Work out the finished part from the listing and answer in its coordinate system (mm). A direction names the side the tool comes from. Coordinates: 2 decimals unless noted, no trailing zeros. Loops run counter-clockwise (first coordinate to the right, second up) from the corner with the lowest first, then second, coordinate; pieces in that order, holes last. Notation, with made-up numbers: M 9,-7.5 L 20,-7.5 A10 cw 20,3.5 Z; hole C 1,78 d9. An arc over 180 degrees is marked long. Write each question's results on one line, items separated by ' | '.
```python
from build123d import *

# Parameters (mm, degrees)
SKETCH1_W              = 25
SKETCH1_H              = 40
BOSS_EXTRUDE1_DEPTH    = 1.6
SKETCH2_W              = 5
SKETCH2_H              = 5
BOSS_EXTRUDE2_DEPTH    = 0.5
SKETCH3_W              = 5
SKETCH3_H              = 3
BOSS_EXTRUDE3_DEPTH    = 2
SKETCH4_R              = 0.95
BOSS_EXTRUDE6_DEPTH    = 2.75
FILLET2_R              = 0.75
LPATTERN2_COUNT        = 3
LPATTERN2_PITCH        = 4
FILLET2_OF_LPATTERN2_R = 0.75
BOSS_EXTRUDE7_DEPTH    = 2.75
SKETCH6_RX             = 1.75
SKETCH6_RY             = 1
BOSS_EXTRUDE8_DEPTH    = 3.5
SKETCH7_W              = 8
SKETCH7_H              = 8
SKETCH7_W_2            = 2.174963518
SKETCH7_H_2            = 1.544625232
SKETCH7_W_3            = 2.304661065
SKETCH7_H_3            = 2.304661065
SKETCH7_W_4            = 1.577304609
SKETCH7_H_4            = 2.386179735
BOSS_EXTRUDE9_DEPTH    = 0.1
SKETCH8_W              = 2.304661065
SKETCH8_H              = 2.304661065
SKETCH8_W_2            = 1.577304609
SKETCH8_H_2            = 2.386179735
SKETCH8_W_3            = 2.174963518
SKETCH8_H_3            = 1.544625232
BOSS_EXTRUDE10_DEPTH   = 1
SKETCH9_W              = 2.75
SKETCH9_H              = 7
BOSS_EXTRUDE11_DEPTH   = 1.5
SKETCH10_W             = 3
SKETCH10_H             = 1
BOSS_EXTRUDE12_DEPTH   = 5
LPATTERN3_COUNT        = 2
LPATTERN3_PITCH        = 17
SKETCH11_W             = 0.854141563
SKETCH11_H             = 2.134375226
BOSS_EXTRUDE13_DEPTH   = 5
CUT_EXTRUDE1_REACH     = 51.369
SKETCH12_R             = 1


with BuildPart() as part:
    # Sketch1 → Boss-Extrude1 (new body)
    with BuildSketch(Plane(origin=(0, 0, 0), x_dir=(1, 0, 0), z_dir=(0, 1, 0))):
        with Locations((12.5, 20)):
            Rectangle(SKETCH1_W, SKETCH1_H)
    extrude(amount=BOSS_EXTRUDE1_DEPTH)

    # Sketch2 → Boss-Extrude2 (add)
    with BuildSketch(Plane(origin=(0, 1.6, 0), x_dir=(1, 0, 0), z_dir=(0, 1, 0))):
        with Locations((12.441080564, 20)):
            Rectangle(SKETCH2_W, SKETCH2_H)
    extrude(amount=BOSS_EXTRUDE2_DEPTH)

    # Sketch3 → Boss-Extrude3 (add)
    with BuildSketch(Plane(origin=(0, 1.6, 0), x_dir=(1, 0, 0), z_dir=(0, 1, 0))):
        with Locations((21.75, 17)):
            Rectangle(SKETCH3_W, SKETCH3_H)
    boss_extrude3 = extrude(amount=BOSS_EXTRUDE3_DEPTH)

    # Sketch4 → Boss-Extrude6 (add)
    with BuildSketch(Plane(origin=(24.25, 0, 0), x_dir=(0, 0, -1), z_dir=(1, 0, 0))):
        with Locations(Location((17, 2.6, 0), (0, 0, 180))):
            Circle(SKETCH4_R)
    boss_extrude6 = extrude(amount=BOSS_EXTRUDE6_DEPTH)

    # Fillet2
    fillet2_edges = [part.edges().sort_by_distance(p)[0] for p in [
        (27, 2.6, -17.95),
    ]]
    fillet(fillet2_edges, radius=FILLET2_R)

    # LPattern2: Boss-Extrude3, Boss-Extrude6 ×3
    with Locations(*[(0, 0, -i * LPATTERN2_PITCH) for i in range(1, LPATTERN2_COUNT)]):
        add(boss_extrude3)
        add(boss_extrude6)

    # Fillet2 of LPattern2
    fillet2_of_lpattern2_edges = [part.edges().sort_by_distance(p)[0] for p in [
        (27, 2.6, -21.95),
        (27, 2.6, -25.95),
    ]]
    fillet(fillet2_of_lpattern2_edges, radius=FILLET2_OF_LPATTERN2_R)

    # Sketch5 → Boss-Extrude7 (add)
    with BuildSketch(Plane(origin=(0, 1.6, 0), x_dir=(1, 0, 0), z_dir=(0, 1, 0))):
        Polygon((24, 30.5), (24, 30), (19, 30), (19, 35), (24, 35), (24, 34.5), (25, 34.5), (25, 30.5), align=None)
    extrude(amount=BOSS_EXTRUDE7_DEPTH)

    # Sketch6 → Boss-Extrude8 (add)
    with BuildSketch(Plane(origin=(25, 0, 0), x_dir=(0, 0, -1), z_dir=(1, 0, 0))):
        with Locations(Location((32.5, 2.975), (0, 0, 180))):
            Ellipse(SKETCH6_RX, SKETCH6_RY)
    extrude(amount=BOSS_EXTRUDE8_DEPTH)

    # Sketch7 → Boss-Extrude9 (add)
    # profile 1 of 4: a face of its own
    with BuildSketch(Plane(origin=(0, 1.6, 0), x_dir=(1, 0, 0), z_dir=(0, 1, 0))):
        with Locations((12.5, 35)):
            Rectangle(SKETCH7_W, SKETCH7_H)
        with Locations((15.249590998, 37.749590998)):
            Rectangle(SKETCH7_W_2, SKETCH7_H_2, mode=Mode.SUBTRACT)
        with Locations((10.522721618, 36.977278383)):
            Rectangle(SKETCH7_W_3, SKETCH7_H_3, mode=Mode.SUBTRACT)
        with Locations((12.965958092, 34.534041908)):
            Rectangle(SKETCH7_W_4, SKETCH7_H_4, mode=Mode.SUBTRACT)
    # profile 2 of 4: a face of its own
    with BuildSketch(Plane(origin=(0, 1.6, 0), x_dir=(1, 0, 0), z_dir=(0, 1, 0))):
        with Locations((15.249590998, 37.749590998)):
            Rectangle(SKETCH7_W_2, SKETCH7_H_2)
    # profile 3 of 4: a face of its own
    with BuildSketch(Plane(origin=(0, 1.6, 0), x_dir=(1, 0, 0), z_dir=(0, 1, 0))):
        with Locations((10.522721618, 36.977278383)):
            Rectangle(SKETCH7_W_3, SKETCH7_H_3)
    # profile 4 of 4: a face of its own
    with BuildSketch(Plane(origin=(0, 1.6, 0), x_dir=(1, 0, 0), z_dir=(0, 1, 0))):
        with Locations((12.965958092, 34.534041908)):
            Rectangle(SKETCH7_W_4, SKETCH7_H_4)
    extrude(amount=BOSS_EXTRUDE9_DEPTH)

    # Sketch8 → Boss-Extrude10 (add)
    with BuildSketch(Plane(origin=(0, 1.7, 0), x_dir=(1, 0, 0), z_dir=(0, 1, 0))):
        with Locations((10.522721618, 36.977278383)):
            Rectangle(SKETCH8_W, SKETCH8_H)
        with Locations((12.965958092, 34.534041908)):
            Rectangle(SKETCH8_W_2, SKETCH8_H_2)
        with Locations((15.249590998, 37.749590998)):
            Rectangle(SKETCH8_W_3, SKETCH8_H_3)
    extrude(amount=BOSS_EXTRUDE10_DEPTH)

    # Sketch9 → Boss-Extrude11 (add)
    with BuildSketch(Plane(origin=(0, 1.6, 0), x_dir=(1, 0, 0), z_dir=(0, 1, 0))):
        with Locations((5.575, 17.5)):
            Rectangle(SKETCH9_W, SKETCH9_H)
    extrude(amount=BOSS_EXTRUDE11_DEPTH)

    # Sketch10 → Boss-Extrude12 (add)
    with BuildSketch(Plane(origin=(0, 1.6, 0), x_dir=(1, 0, 0), z_dir=(0, 1, 0))):
        Polygon((6.4, 13), (0.4, 13), (0.4, 5), (6.4, 5), (6.4, 7), (5.9, 7), (5.9, 11), (6.4, 11), align=None)
        with Locations((3.4, 11.5)):
            Rectangle(SKETCH10_W, SKETCH10_H, mode=Mode.SUBTRACT)
        with Locations((3.4, 6.5)):
            Rectangle(SKETCH10_W, SKETCH10_H, mode=Mode.SUBTRACT)
    boss_extrude12 = extrude(amount=BOSS_EXTRUDE12_DEPTH)

    # LPattern3: Boss-Extrude12 ×2
    with Locations(*[(0, 0, -i * LPATTERN3_PITCH) for i in range(1, LPATTERN3_COUNT)]):
        add(boss_extrude12)

    # Sketch11 → Boss-Extrude13 (add)
    with BuildSketch(Plane(origin=(0, 1.6, 0), x_dir=(1, 0, 0), z_dir=(0, 1, 0))):
        Polygon((7.3, 39.6), (0.4, 39.6), (0.4, 34.9), (1.524996245, 34.9), (1.524996245, 35.4), (6.175003755, 35.4), (6.175003755, 34.9), (7.3, 34.9), align=None)
        with Locations((5.747932974, 37.25)):
            Rectangle(SKETCH11_W, SKETCH11_H, mode=Mode.SUBTRACT)
        with Locations((1.952067027, 37.25)):
            Rectangle(SKETCH11_W, SKETCH11_H, mode=Mode.SUBTRACT)
    extrude(amount=BOSS_EXTRUDE13_DEPTH)

    # Sketch12 → Cut-Extrude1 (cut, up to next)
    with BuildSketch(Plane(origin=(0, 1.6, 0), x_dir=(1, 0, 0), z_dir=(0, 1, 0)), mode=Mode.PRIVATE) as cut_extrude1_sk1:
        with Locations(Location((3.5, 2.5, 0), (0, 0, 270))):
            Circle(SKETCH12_R)
    cut_extrude1_tool1 = extrude(cut_extrude1_sk1.sketch, amount=-CUT_EXTRUDE1_REACH, mode=Mode.PRIVATE) & part.part
    # Sketch12 → Cut-Extrude1 (cut, up to next)
    with BuildSketch(Plane(origin=(0, 1.6, 0), x_dir=(1, 0, 0), z_dir=(0, 1, 0)), mode=Mode.PRIVATE) as cut_extrude1_sk2:
        with Locations(Location((21.5, 2.5, 0), (0, 0, 270))):
            Circle(SKETCH12_R)
    cut_extrude1_tool2 = extrude(cut_extrude1_sk2.sketch, amount=-CUT_EXTRUDE1_REACH, mode=Mode.PRIVATE) & part.part
    # Sketch12 → Cut-Extrude1 (cut, up to next)
    with BuildSketch(Plane(origin=(0, 1.6, 0), x_dir=(1, 0, 0), z_dir=(0, 1, 0)), mode=Mode.PRIVATE) as cut_extrude1_sk3:
        with Locations(Location((21.5, 37.5, 0), (0, 0, 270))):
            Circle(SKETCH12_R)
    cut_extrude1_tool3 = extrude(cut_extrude1_sk3.sketch, amount=-CUT_EXTRUDE1_REACH, mode=Mode.PRIVATE) & part.part
    add(cut_extrude1_tool1.solids().sort_by_distance((3.5, 1.6, -2.5))[0], mode=Mode.SUBTRACT)
    add(cut_extrude1_tool2.solids().sort_by_distance((21.5, 1.6, -2.5))[0], mode=Mode.SUBTRACT)
    add(cut_extrude1_tool3.solids().sort_by_distance((21.5, 1.6, -37.5))[0], mode=Mode.SUBTRACT)


solid = part.part
```
1) Find section D-D, the plane x = 11.25. Give the vertices of the cut face in (y, z), and give its area (3 significant figures).
Check result:
outline: M 0,-40 L 1.6,-40 L 1.6,-39 L 1.7,-39 L 1.7,-38.13 L 2.7,-38.13 L 2.7,-35.82 L 1.7,-35.82 L 1.7,-31 L 1.6,-31 L 1.6,-22.5 L 2.1,-22.5 L 2.1,-17.5 L 1.6,-17.5 L 1.6,0 L 0,0 Z | area: 69.6 mm^2
2) Which of the six approach directions +Z, -Z, +X, -X, +Y, -Y give full straight-line access (tool end or side, diameter ignored) to faces 4 (the face through (4.9, 4.1, -11.5)), 5 (the face through (24.5, 3, -30.5)), 6 (the face through (19, 3, -32)), 7 (the face through (12, 2.1, -20)), 8 (the face through (3, 4, -13))?
Check result:
face 4: +Y | face 5: +X, +Y | face 6: +Z, -Z, +Y | face 7: +Z, +Y | face 8: +X, -X, +Y
3) Given pin 1 Ø3 at (y, z) = (3.5, -28.5) entering from -X; pin 2 Ø3.5 at (x, y) = (3.5, 4) entering from +Z; pin 3 Ø0.6 at (y, z) = (5.5, -11.5) entering from +X, each flat-ended and moving along its own axis, determine where each tip first touches the part or whether it passes through.
Check result:
pin 1: x = 0.4 | pin 2: z = -5 | pin 3: x = 6.4
4) Find section A-A, the plane x = 21.5. Give the vertices of the cut face in (y, z), and give its area (4 significant figures).
Check result:
outline: M 0,-40 L 1.6,-40 L 1.6,-38.5 L 0,-38.5 Z; M 0,-36.5 L 1.6,-36.5 L 1.6,-35 L 4.35,-35 L 4.35,-30 L 1.6,-30 L 1.6,-26.5 L 3.6,-26.5 L 3.6,-23.5 L 1.6,-23.5 L 1.6,-22.5 L 3.6,-22.5 L 3.6,-19.5 L 1.6,-19.5 L 1.6,-18.5 L 3.6,-18.5 L 3.6,-15.5 L 1.6,-15.5 L 1.6,-3.5 L 0,-3.5 Z; M 0,-1.5 L 1.6,-1.5 L 1.6,0 L 0,0 Z | area: 89.35 mm^2
5) Straight lines are drawn through the part: probe 1 along X at (y, z) = (0.95, -2.5); probe 2 along X at (y, z) = (1.2, -37.5); probe 3 along Z at (x, y) = (21.25, 2.25). For each, find the intervals that lie inside material, in ascending order. Write a range as [from, to].
Check result:
probe 1: [0, 2.5], [4.5, 20.5], [22.5, 25] | probe 2: [0, 20.5], [22.5, 25] | probe 3: [-35, -30], [-26.5, -23.5], [-22.5, -19.5], [-18.5, -15.5]
6) For a pull along Z with two mould halves and no side action, classify faces 1 (the face through (22, 3, -15.5)), 2 (the face through (1.9, 4.1, -6.5)), 3 (the face through (22, 3.6, -25)) as released by +Z, released by -Z, zero draft, split by the parting line, or undercut.
Check result:
face 1: released by +Z | face 2: undercut | face 3: zero draft
7) Find section C-C, the plane y = 5.5. Give the number of separate pieces and of enclosed holes in the cut face, and give its area (3 significant figures).
Check result:
separate pieces: 3 | enclosed holes: 6 | area: 106 mm^2
